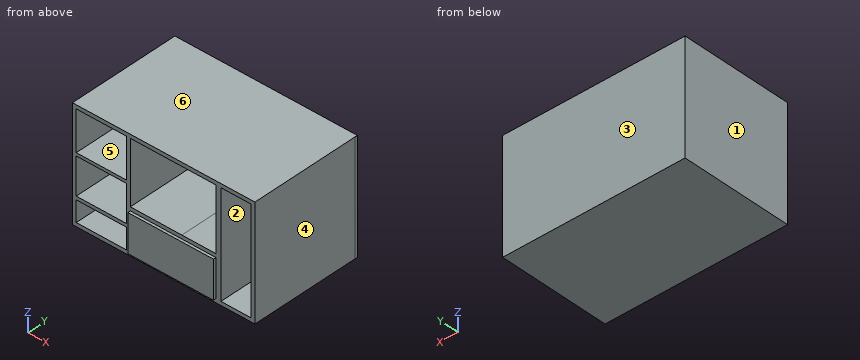
```python
from build123d import *

# Parameters (mm, degrees)
F0_W      = 1841.5
F0_H      = 1130.3
F1_DEPTH  = 1130.3
F3_W      = 1827.532351
F3_H      = 1129.572153
F4_DEPTH  = 25.4
F5_W      = 865.357041
F5_H      = 376.358599
F6_DEPTH  = 25.4
F7_W      = 831.391633
F7_H      = 382.297545
F8_DEPTH  = 25.4
F9_W      = 863.6
F9_H      = 381
F10_DEPTH = 1131.859899


with BuildPart() as f1:
    # F0 (on Front) → F1 (new body)
    with BuildSketch(Plane.XZ):
        Rectangle(F0_W, F0_H)
        Polygon((882.65, 527.05), (882.65, -527.05), (577.85, -527.05), (527.05, -527.05), (-336.55, -527.05), (-374.65, -527.05), (-882.65, -527.05), (-882.65, -316.212654), (-882.65, -282.136858), (-882.65, 89.881361), (-882.65, 120.749831), (-882.65, 527.05), (-374.65, 527.05), (-336.55, 527.05), (527.05, 527.05), (577.85, 527.05), align=None, mode=Mode.SUBTRACT)
        Polygon((-374.65, -527.05), (-336.55, -527.05), (-336.55, -146.05), (-336.55, -107.95), (-336.55, 0), (-336.55, 527.05), (-374.65, 527.05), (-374.65, 120.749831), (-374.65, 89.881361), (-374.65, -120.674253), (-374.65, -282.136858), (-374.65, -316.212654), align=None)
        Polygon((-374.65, 89.881361), (-374.65, 120.749831), (-752.773166, 120.749831), (-882.65, 120.749831), (-882.65, 89.881361), (-408.513486, 89.881361), align=None)
        Polygon((-882.65, -316.212654), (-374.65, -316.212654), (-374.65, -282.136858), (-408.513486, -282.136858), (-882.65, -282.136858), align=None)
        Polygon((-336.55, -107.95), (-336.55, -146.05), (182.885635, -147.757417), (182.885635, -109.657417), align=None)
        Polygon((182.885635, -147.757417), (527.05, -148.888707), (527.05, -109.657417), (182.885635, -109.657417), align=None)
        Polygon((527.05, -527.05), (577.85, -527.05), (577.85, -145.718575), (577.85, 527.05), (527.05, 527.05), (527.05, -109.657417), (527.05, -148.888707), align=None)
    extrude(amount=F1_DEPTH)

    # F3 (on face) → F4 (join)
    with BuildSketch(Plane.XZ):
        with Locations((8.99306, -0.142456)):
            Rectangle(F3_W, F3_H)
    extrude(amount=F4_DEPTH)

    # F5 (on face) → F6 (join)
    with BuildSketch(Plane.XZ.offset(25.4)):
        with Locations((94.785392, -343.243077)):
            Rectangle(F5_W, F5_H)
    extrude(amount=-F6_DEPTH)

    # F7 (on face) → F8 (join)
    with BuildSketch(Plane.XZ.offset(25.4)):
        with Locations((134.62612, -372.283206)):
            Rectangle(F7_W, F7_H)
    extrude(amount=-F8_DEPTH)

    # F9 (on face) → F10 (join)
    with BuildSketch(Plane.XZ.offset(25.4)):
        with Locations((95.25, -336.55)):
            Rectangle(F9_W, F9_H)
    extrude(amount=F10_DEPTH)


solid = f1.part
```
Input: part model. Units: mm. Frame: model coordinates. Face numbers are marked on the shaded views. A direction names the side the tool comes from. Round coordinates to 2 decimals unless told otherwise and drop trailing zeros. Write each loop counter-clockwise with the first axis right and the second up, starting at its lowest first coordinate (ties: lowest second). Pieces come first, ordered by that corner, then holes. Notation, with made-up numbers: (-6, 26.25) -> (15, 26.25) arc R12 ccw to (15, 49.25) -> close; hole circle Ø11 at (12, 19). An arc over 180 degrees is marked (long way). Answer as CSV lines item,"result".
1. Section B-B (y = -745). Return the cut outline in (x, z).
Geometry says:
outline,"(-920.75, -565.15) -> (920.75, -565.15) -> (920.75, 565.15) -> (-920.75, 565.15) -> close; hole (-882.65, -527.05) -> (-374.65, -527.05) -> (-374.65, -316.21) -> (-882.65, -316.21) -> close; hole (-882.65, -282.14) -> (-374.65, -282.14) -> (-374.65, 89.88) -> (-882.65, 89.88) -> close; hole (-882.65, 120.75) -> (-374.65, 120.75) -> (-374.65, 527.05) -> (-882.65, 527.05) -> close; hole (-336.55, -107.95) -> (182.89, -109.66) -> (527.05, -109.66) -> (527.05, 527.05) -> (-336.55, 527.05) -> close; hole (577.85, -527.05) -> (882.65, -527.05) -> (882.65, 527.05) -> (577.85, 527.05) -> close"
2. Ray query, L1, parallel to X at y = -857, z = -510; L2, parallel to X at y = -354, z = 90; L3, parallel to X at y = -692, z = 475.5. Return the intervals inside material, ascending. Write a range as [from, to].
Geometry says:
L1,"x = [-920.75, -882.65], [-374.65, 577.85], [882.65, 920.75]"
L2,"x = [-920.75, -336.55], [527.05, 577.85], [882.65, 920.75]"
L3,"x = [-920.75, -882.65], [-374.65, -336.55], [527.05, 577.85], [882.65, 920.75]"
3. Section D-D (x = -589). Return the cut outline in (y, z), plus the area to 3 significant figures.
Geometry says:
outline,"(-1130.3, -565.15) -> (0, -565.15) -> (0, 565.15) -> (-1130.3, 565.15) -> (-1130.3, 527.05) -> (-25.4, 527.05) -> (-25.4, 120.75) -> (-1130.3, 120.75) -> (-1130.3, 89.88) -> (-25.4, 89.88) -> (-25.4, -282.14) -> (-1130.3, -282.14) -> (-1130.3, -316.21) -> (-25.4, -316.21) -> (-25.4, -527.05) -> (-1130.3, -527.05) -> close"
area,"185,000 mm^2"
4. Contact query for flat-ended pins moving along their axis: P1, Ø0.6, axis at x = 922, z = 268, coming from the -Y side; P2, Ø1.5, axis at y = -502.5, z = -105.5, coming from the +X side; P3, Ø1.6, axis at x = 921.5, y = -12, coming from the +Z side; P4, Ø8, axis at y = -1144.5, z = -344.5, coming from the +X side. Output: stop coordinate, or through.
Geometry says:
P1,"stops at y = -25.4"
P2,"stops at x = 920.75"
P3,"stops at z = 565.15"
P4,"stops at x = 527.05"
5. Section C-C (x = 335). Return the cut outline in (y, z).
Geometry says:
outline,"(-1157.26, -527.05) -> (-1130.3, -527.05) -> (-1130.3, -565.15) -> (0, -565.15) -> (0, 565.15) -> (-1130.3, 565.15) -> (-1130.3, 527.05) -> (-25.4, 527.05) -> (-25.4, -109.66) -> (-1130.3, -109.66) -> (-1130.3, -146.05) -> (-1157.26, -146.05) -> close"
6. Reachability of the marked faces 5 and 6 from +Z, -Z, +X, -X, +Y, -Y: full face, straight path, thin tool, end or side. Return the list, or none.
Geometry says:
face 5,"-Y"
face 6,"+Z, +X, -X, +Y, -Y"
7. Mould query, pull axis X, two halves, no side actions, for the marked faces 1, 2, 3 and 4. Classes: +X half, -X half, draft (parallel to the pull), parting line (faces both ways), or undercut.
Geometry says:
face 1,"-X half"
face 2,"undercut"
face 3,"draft"
face 4,"+X half"
8. Section A-A (z = 255.5). Return the cut outline in (x, y).
Geometry says:
outline,"(-920.75, -1130.3) -> (-882.65, -1130.3) -> (-882.65, -25.4) -> (-374.65, -25.4) -> (-374.65, -1130.3) -> (-336.55, -1130.3) -> (-336.55, -25.4) -> (527.05, -25.4) -> (527.05, -1130.3) -> (577.85, -1130.3) -> (577.85, -25.4) -> (882.65, -25.4) -> (882.65, -1130.3) -> (920.75, -1130.3) -> (920.75, -25.4) -> (922.76, -25.4) -> (922.76, 0) -> (-920.75, 0) -> close"
